from build123d import *

# Parameters (mm, degrees)
BOSS_EXTRUDE1_DEPTH = 25
SKETCH2_R           = 2.1
CUT_EXTRUDE1_DEPTH  = 72.589105316
CUT_EXTRUDE2_DEPTH  = 10


with BuildPart() as part:
    # Sketch1 → Boss-Extrude1 (new body)
    with BuildSketch(Plane.XY):
        with BuildLine():
            Line((-30, 0), (-20, 0))
            ThreePointArc((-20, 0), (0, 20), (20, 0))
            Line((20, 0), (30, 0))
            Line((30, 0), (30, 30))
            Line((30, 30), (-30, 30))
            Line((-30, 30), (-30, 0))
        make_face()
        with BuildLine():
            ThreePointArc((20, 0), (0, -20), (-20, 0))
            Line((-20, 0), (-30, 0))
            Line((-30, 0), (-30, -30))
            Line((-30, -30), (30, -30))
            Line((30, -30), (30, 0))
            Line((30, 0), (20, 0))
        make_face()
    extrude(amount=BOSS_EXTRUDE1_DEPTH)

    # Sketch2 → Cut-Extrude1 (cut, through all)
    with BuildSketch(Plane(origin=(30, 0, 0), x_dir=(0, 0, -1), z_dir=(1, 0, 0))):
        with Locations((-12.5, 25)):
            Circle(SKETCH2_R)
        with Locations((-12.5, -25)):
            Circle(SKETCH2_R)
        with Locations((-12.5, 0)):
            Circle(SKETCH2_R)
    extrude(amount=-CUT_EXTRUDE1_DEPTH, mode=Mode.SUBTRACT)

    # Sketch3 → Cut-Extrude2 (cut)
    with BuildSketch(Plane(origin=(0, 30, 0), x_dir=(1, 0, 0), z_dir=(0, 1, 0))):
        Polygon((-30, -18.5), (-23, -18.5), (-23, -15), (-23, -10), (-23, -6.5), (-30, -6.5), align=None)
        Polygon((23, -10), (23, -15), (23, -18.5), (30, -18.5), (30, -6.5), (23, -6.5), align=None)
    cut_extrude2 = extrude(amount=-CUT_EXTRUDE2_DEPTH, mode=Mode.SUBTRACT)

    # Mirror1: Cut-Extrude2 across plane
    add(cut_extrude2.mirror(Plane.ZX), mode=Mode.SUBTRACT)


solid = part.part
Verification items for the finished model (mm, model axes). A direction names the side the tool comes from. Round coordinates to 2 decimals unless told otherwise and drop trailing zeros. Loops run counter-clockwise (first coordinate to the right, second up) from the corner with the lowest first, then second, coordinate; pieces in that order, holes last. Notation, with made-up numbers: (86.5, 20.25) - (94.5, 20.25) arc R23 cw to (94.5, 42.25) - close; hole circle Ø8 at (48.5, 58.5). An arc over 180 degrees is marked (long way). Use a Markdown table: item, result. Add a question column.
1. Section check C-C, the plane z = 12.5. Record the boundary of the cut face in (x, y), plus the area to 3 significant figures.
2. Thickness scan on probe 1 along Y at (x, z) = (-21.75, 12.5); probe 2 along Y at (x, z) = (0, 6.25); probe 3 along Y at (x, z) = (5, 11.5). Record the ranges inside material, lowest first. Write a range as [from, to].
3. Gauge pin test, flat ends, axial feed: pin 1 (8 mm diameter, centred on y = 24.5, z = 13, fed in from -X); pin 2 (3.5 mm diameter, centred on x = 25.5, z = 14, fed in from -Y); pin 3 (3 mm diameter, centred on y = -25.5, z = 12.5, fed in from +X). Record the tip position at first contact, or that the pin passes through.
4. Section check D-D, the plane y = -25. Record the boundary of the cut face in (x, z).
5. Section check A-A, the plane x = 0. Record the boundary of the cut face in (y, z).
6. Release check for a two-part mould opening along Z. For faces 1 (the face through (-0.4, 20.4, 0)), 2 (the face through (-30, 0, 10)), 3 (the face through (27, 25, 6.5)) record: released by +Z, released by -Z, zero draft, split by the parting line, or undercut.
7. Access from +Z, -Z, +X, -X, +Y, -Y to the whole of each face (thin tool, end or side, straight path). Record for faces 4 (the face through (-27, -25, 18.5)), 5 (the face through (26, 20, 12)), 6 (the face through (27, -25, 6.5)).
8. Section check B-B, the plane y = 0. Record the boundary of the cut face in (x, z), plus the area to 3 significant figures.
Checks:
| question | item | result |
|---|---|---|
| 1 | outline | (-30, -20) - (-23, -20) - (-23, -22.9) - (23, -22.9) - (23, -20) - (30, -20) - (30, -2.1) - (19.89, -2.1) arc R20 cw to (-19.89, -2.1) - (-30, -2.1) - close; (-30, 2.1) - (-19.89, 2.1) arc R20 cw to (19.89, 2.1) - (30, 2.1) - (30, 20) - (23, 20) - (23, 22.9) - (-23, 22.9) - (-23, 20) - (-30, 20) - close; (-23, -30) - (23, -30) - (23, -27.1) - (-23, -27.1) - close; (-23, 27.1) - (23, 27.1) - (23, 30) - (-23, 30) - close |
| 1 | area | 1,590 mm^2 |
| 2 | probe 1 | y = [-30, -27.1], [-22.9, -2.1], [2.1, 22.9], [27.1, 30] |
| 2 | probe 2 | y = [-30, -20], [20, 30] |
| 2 | probe 3 | y = [-30, -26.85], [-23.15, -19.36], [19.36, 23.15], [26.85, 30] |
| 3 | pin 1 | stops at x = -23 |
| 3 | pin 2 | stops at y = -20 |
| 3 | pin 3 | passes through |
| 4 | outline | (-30, 0) - (30, 0) - (30, 6.5) - (23, 6.5) - (23, 10.4) - (-23, 10.4) - (-23, 6.5) - (-30, 6.5) - close; (-30, 18.5) - (-23, 18.5) - (-23, 14.6) - (23, 14.6) - (23, 18.5) - (30, 18.5) - (30, 25) - (-30, 25) - close |
| 5 | outline | (-30, 0) - (-20, 0) - (-20, 25) - (-30, 25) - close; (20, 0) - (30, 0) - (30, 25) - (20, 25) - close; hole circle Ø4.2 at (-25, 12.5); hole circle Ø4.2 at (25, 12.5) |
| 6 | face 1 | released by -Z |
| 6 | face 2 | zero draft |
| 6 | face 3 | undercut |
| 7 | face 4 | -X, -Y |
| 7 | face 5 | +X, +Y |
| 7 | face 6 | +X, -Y |
| 8 | outline | (-30, 0) - (-20, 0) - (-20, 10.4) - (-30, 10.4) - close; (-30, 14.6) - (-20, 14.6) - (-20, 25) - (-30, 25) - close; (20, 0) - (30, 0) - (30, 10.4) - (20, 10.4) - close; (20, 14.6) - (30, 14.6) - (30, 25) - (20, 25) - close |
| 8 | area | 416 mm^2 |
